Here's how the part is built. I have some questions about the finished solid (model axes, mm). Face numbers are marked on the shaded views. Round coordinates to 2 decimals unless told otherwise and drop trailing zeros. Put each result on its own line as item: value. Start each with the question number.
1) If I drill on line 1 along X through (y, z) = (-2.5, 40); line 2 along Z through (x, y) = (-61, -0.9); line 3 along X through (y, z) = (-0.2, -38.5), over which ranges is the centre line in solid material (lowest first)? Write a range as [from, to].
2) Will these pins go through, and if not, where does the flat tip stop? P1, Ø10, axis at x = -51.5, z = 32, coming from the +Y side; P2, Ø5, axis at x = -58.68, z = 37.55, coming from the -Y side.
3) We'd pull the mould along Y, two halves only. Please class the marked faces 1 and 2: released by +Y, released by -Y, zero draft, split by the parting line, or undercut.
from build123d import *

# Parameters (mm, degrees)
F0_W     = 136.5267336369
F0_H     = 88.4205549955
F1_DEPTH = 3
F2_D     = 30
F3_W     = 117.3540726304
F3_H     = 75.1073509455
F4_DEPTH = 3
F5_D     = 6
F6_D     = 3


with BuildPart() as f1:
    # F0 (on Front) → F1 (new body)
    with BuildSketch(Plane.XZ):
        Rectangle(F0_W, F0_H)
    extrude(amount=F1_DEPTH)

    # F2 (through all)
    with Locations(Plane(origin=(0, 0, 0), x_dir=(1, 0, 0), z_dir=(0, 1, 0))):
        with Locations((0, 0)):
            Hole(F2_D / 2)

    # F3 (on Front) → F4 (join)
    with BuildSketch(Plane.XZ):
        Rectangle(F3_W, F3_H)
    extrude(amount=F4_DEPTH)

    # F5 (through all)
    with Locations(Plane(origin=(0, 0, 0), x_dir=(1, 0, 0), z_dir=(0, 1, 0))):
        with Locations((-58.6770363152, -37.5536754727)):
            Hole(F5_D / 2)

    # F6 (through all)
    with Locations(Plane(origin=(0, 0, 0), x_dir=(1, 0, 0), z_dir=(0, 1, 0))):
        with Locations((-58.6770363152, 37.5536754727), (-58.6770363152, -37.5536754727)):
            Hole(F6_D / 2)


solid = f1.part
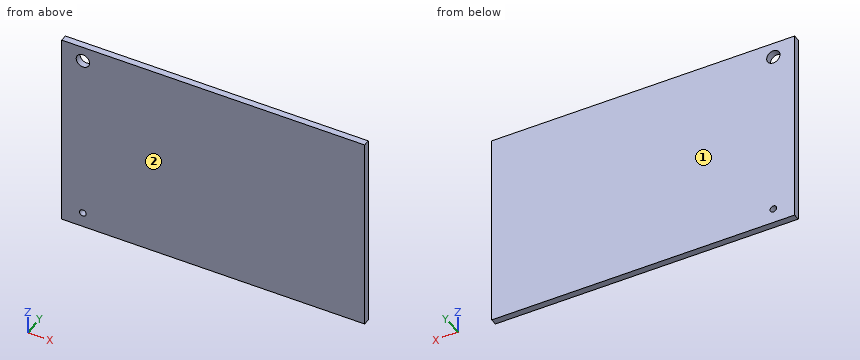
Findings:
1. line 1: x = [-68.26, -60.41], [-56.94, 68.26]
1. line 2: z = [-44.21, 35.66], [39.45, 44.21]
1. line 3: x = [-68.26, -59.84], [-57.51, 68.26]
2. P1: stops at y = 0
2. P2: passes through
3. face 1: released by +Y
3. face 2: released by -Y
